```python
from build123d import *

# Parameters (mm, degrees)
SKETCH_W        = 22
SKETCH_H        = 26
PAD_DEPTH       = 2
SKETCH007_W     = 10
SKETCH007_H     = 5
POCKET_DEPTH    = 2.001
SKETCH008_W     = 22
SKETCH008_H     = 26
SKETCH008_W_2   = 14
SKETCH008_H_2   = 16
PAD005_DEPTH    = 46
SKETCH009_W     = 18.2
SKETCH009_H     = 16
POCKET002_DEPTH = 41.5
SKETCH010_W     = 18.2
SKETCH010_H     = 1.4
POCKET003_DEPTH = 4.5
SKETCH013_R     = 1.5
POCKET005_DEPTH = 5
FILLET001_R     = 1


with BuildPart() as part:
    # Sketch → Pad (new body)
    with BuildSketch(Plane.XY):
        Rectangle(SKETCH_W, SKETCH_H)
    extrude(amount=PAD_DEPTH)

    # Sketch007 (on Face6 of Pad) → Pocket (cut, through all)
    with BuildSketch(Plane.XY.offset(2)):
        with Locations((0, 2.5)):
            Rectangle(SKETCH007_W, SKETCH007_H)
    extrude(amount=-POCKET_DEPTH, mode=Mode.SUBTRACT)

    # Sketch008 (on Face5 of Pocket) → Pad005 (join)
    with BuildSketch(Plane.XY.offset(2)):
        Rectangle(SKETCH008_W, SKETCH008_H)
        Rectangle(SKETCH008_W_2, SKETCH008_H_2, mode=Mode.SUBTRACT)
    extrude(amount=PAD005_DEPTH)

    # Sketch009 (on Face13 of Pad005) → Pocket002 (cut)
    with BuildSketch(Plane.XY.offset(48)):
        Rectangle(SKETCH009_W, SKETCH009_H)
    extrude(amount=-POCKET002_DEPTH, mode=Mode.SUBTRACT)

    # Sketch010 (on Face29 of Pocket002) → Pocket003 (cut)
    with BuildSketch(Plane.XY.offset(6.5)):
        Rectangle(SKETCH010_W, SKETCH010_H)
    extrude(amount=-POCKET003_DEPTH, mode=Mode.SUBTRACT)

    # Sketch013 (on Face13 of Pocket003) → Pocket005 (cut)
    with BuildSketch(Plane.XY.offset(48)):
        with Locations((0, 10.5)):
            Circle(SKETCH013_R)
        with Locations((0, -10.5)):
            Circle(SKETCH013_R)
    extrude(amount=-POCKET005_DEPTH, mode=Mode.SUBTRACT)

    # Fillet001
    fillet001_edges = [part.edges().sort_by_distance(p)[0] for p in [
        (-11, 13, 25),
        (-11, -13, 25),
        (11, 13, 25),
        (11, -13, 25),
        (11, -13, 1),
        (11, 13, 1),
        (-11, 13, 1),
        (-11, -13, 1),
    ]]
    fillet(fillet001_edges, radius=FILLET001_R)


solid = part.part
```
Here's how the part is built. I have some questions about the finished solid (model axes, mm). A direction names the side the tool comes from. Coordinates: 2 decimals unless noted, no trailing zeros. Write each loop counter-clockwise with the first axis right and the second up, starting at its lowest first coordinate (ties: lowest second). Pieces come first, ordered by that corner, then holes. Notation, with made-up numbers: (67, -29.75) -> (103, -29.75) arc R25 cw to (103, -0.75) -> close; hole circle Ø10 at (80, 4). An arc over 180 degrees is marked (long way). Use a Markdown table: item, result. Add a question column.
(1) For faces 1 (the flat face through (0, -3, 0)), 2 (the flat face through (0, 0, 1)), 3 (the flat face through (-8, 4, 6.5)), which set-ups out of +Z, -Z, +X, -X, +Y, -Y let a thin tool reach every point of the face, with its end or its side?
(2) If we section it at C-C, the plane x = -6.5: Write out the boundary of the cut face in (y, z).
(3) If we section it at A-A, the plane x = 0: Write out the boundary of the cut face in (y, z).
(4) If we section it at B-B, the plane z = 19.5: Write out the boundary of the cut face in (x, y).
(5) We'd pull the mould along X, two halves only. Please class faces 4 (the cylindrical face through (10.699, 12.715, 23.664)), 5 (the cylindrical face through (-10.715, 12.699, 23.664)), 6 (the flat face through (0, -8, 25)): +X half, -X half, draft (parallel to the pull), parting line (faces both ways), or undercut.
(6) If we section it at D-D, the plane y = -4.75: Write out the boundary of the cut face in (x, z), and give its area (3 significant figures).
(7) Please list where these lines run through material, in increasing order: line 1 (Y direction, x = 0, z = 46.25); line 2 (Y direction, x = -2.5, z = 16); line 3 (X direction, y = 0.75, z = 28).
(8) I'm going to push flat-ended pins straight in: P1, Ø2.5, axis at x = 0, y = 10.5, coming from the +Z side; P2, Ø0.6, axis at x = 8.5, y = -5, coming from the +Z side; P3, Ø5, axis at x = 2, y = 0.5, coming from the +Z side. Where does each tip first touch, or does it pass through?
Outcome:
| question | item | result |
|---|---|---|
| 1 | face 1 | -Z, +X, -X, +Y, -Y |
| 1 | face 2 | +Z, -Z |
| 1 | face 3 | +Z |
| 2 | outline | (-13, 0) -> (13, 0) -> (13, 48) -> (8, 48) -> (8, 2) -> (-8, 2) -> (-8, 48) -> (-13, 48) -> close |
| 3 | outline | (-13, 0) -> (0, 0) -> (0, 2) -> (-8, 2) -> (-8, 48) -> (-9, 48) -> (-9, 43) -> (-12, 43) -> (-12, 48) -> (-13, 48) -> close; (5, 0) -> (13, 0) -> (13, 48) -> (12, 48) -> (12, 43) -> (9, 43) -> (9, 48) -> (8, 48) -> (8, 2) -> (5, 2) -> close |
| 4 | outline | (-11, -12) arc R1 ccw to (-10, -13) -> (10, -13) arc R1 ccw to (11, -12) -> (11, 12) arc R1 ccw to (10, 13) -> (-10, 13) arc R1 ccw to (-11, 12) -> close; hole (-9.1, -8) -> (9.1, -8) -> (9.1, 8) -> (-9.1, 8) -> close |
| 5 | face 4 | +X half |
| 5 | face 5 | -X half |
| 5 | face 6 | undercut |
| 6 | outline | (-11, 0) -> (11, 0) -> (11, 48) -> (9.1, 48) -> (9.1, 6.5) -> (7, 6.5) -> (7, 2) -> (-7, 2) -> (-7, 6.5) -> (-9.1, 6.5) -> (-9.1, 48) -> (-11, 48) -> close |
| 6 | area | 238 mm^2 |
| 7 | line 1 | y = -13 to -12, -9 to -8, 8 to 9, 12 to 13 |
| 7 | line 2 | y = -13 to -8, 8 to 13 |
| 7 | line 3 | x = -11 to -9.1, 9.1 to 11 |
| 8 | P1 | stops at z = 43 |
| 8 | P2 | stops at z = 6.5 |
| 8 | P3 | stops at z = 2 |
